Geometry check sheet. Reference: the model listing, model coordinates, mm. Face numbers are marked on the shaded views. Give positions to 0.01 mm unless a question says otherwise; leave off trailing zeros. Order: outer loops, then holes, each group sorted by start corner. A loop starts at its lowest first (then second) coordinate and runs counter-clockwise, first axis right, second up.
from build123d import *

# Parameters (mm, degrees)
SKETCH_1_R          = 53
SKETCH_1_R_2        = 45
EXTRUDE_1_DEPTH     = 8
SKETCH_2_R          = 50.25
SKETCH_2_R_2        = 46.75
CUT_EXTRUDE_1_DEPTH = 1
CUT_EXTRUDE_START   = -7
SKETCH_2_2_R        = 50.25
SKETCH_2_2_R_2      = 46.75
CUT_EXTRUDE_2_DEPTH = 1


with BuildPart() as part:
    # 草图1 → 凸台-拉伸1 (new body)
    with BuildSketch(Plane(origin=(0, 0, 0), x_dir=(1, 0, 0), z_dir=(0, 1, 0))):
        with Locations(Location((0, 0, 0), (0, 0, 270))):
            Circle(SKETCH_1_R)
        with Locations(Location((0, 0, 0), (0, 0, 270))):
            Circle(SKETCH_1_R_2, mode=Mode.SUBTRACT)
    extrude(amount=EXTRUDE_1_DEPTH)

    # 草图2 → 切除-拉伸1 (cut)
    with BuildSketch(Plane(origin=(0, 8, 0), x_dir=(1, 0, 0), z_dir=(0, 1, 0))):
        with Locations(Location((0, 0, 0), (0, 0, 270))):
            Circle(SKETCH_2_R)
        with Locations(Location((0, 0, 0), (0, 0, 270))):
            Circle(SKETCH_2_R_2, mode=Mode.SUBTRACT)
    extrude(amount=-CUT_EXTRUDE_1_DEPTH, mode=Mode.SUBTRACT)

    # 草图2<2> → 切除-拉伸2 (cut)
    with BuildSketch(Plane(origin=(0, 8, 0), x_dir=(1, 0, 0), z_dir=(0, 1, 0)).offset(CUT_EXTRUDE_START)):
        with Locations(Location((0, 0, 0), (0, 0, 270))):
            Circle(SKETCH_2_2_R)
        with Locations(Location((0, 0, 0), (0, 0, 270))):
            Circle(SKETCH_2_2_R_2, mode=Mode.SUBTRACT)
    extrude(amount=-CUT_EXTRUDE_2_DEPTH, mode=Mode.SUBTRACT)


solid = part.part
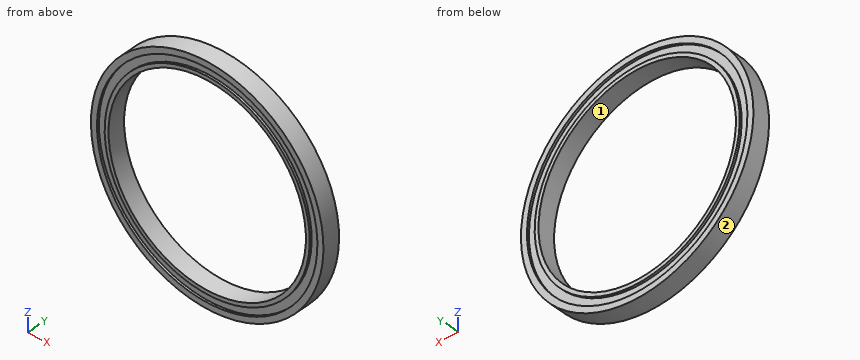
Item 1: Sectioned sample at C-C (y = 2.75). Enter the section's corners in (x, z), and give its area (3 significant figures).
Reported:
outline: circle Ø106 at (0, 0); hole circle Ø90 at (0, 0)
area: 2,460 mm2
Item 2: Sectioned sample at B-B (z = -43). Enter the section's corners in (x, y).
Reported:
outline: (-30.98, 0) - (-26, 0) - (-26, 1) - (-18.35, 1) - (-18.35, 0) - (-13.27, 0) - (-13.27, 8) - (-18.35, 8) - (-18.35, 7) - (-26, 7) - (-26, 8) - (-30.98, 8) - close; (13.27, 0) - (18.35, 0) - (18.35, 1) - (26, 1) - (26, 0) - (30.98, 0) - (30.98, 8) - (26, 8) - (26, 7) - (18.35, 7) - (18.35, 8) - (13.27, 8) - close
Item 3: Draft check along X on the marked faces 1 and 2. Enter one of: released by +X, released by -X, zero draft, split by the parting line, or undercut.
Reported:
face 1: undercut
face 2: split by the parting line
Item 4: Scan lines: L1, parallel to X at y = 0.6, z = 0; L2, parallel to X at y = 6, z = 0; L3, parallel to X at y = 7.75, z = -29.5. Record each from-to range of solid material in increasing order.
Reported:
L1: x = -53 to -50.25, -46.75 to -45, 45 to 46.75, 50.25 to 53
L2: x = -53 to -45, 45 to 53
L3: x = -44.03 to -40.68, -36.27 to -33.98, 33.98 to 36.27, 40.68 to 44.03
Item 5: Sectioned sample at A-A (x = 0). Enter the section's corners in (y, z).
Reported:
outline: (0, -53) - (8, -53) - (8, -50.25) - (7, -50.25) - (7, -46.75) - (8, -46.75) - (8, -45) - (0, -45) - (0, -46.75) - (1, -46.75) - (1, -50.25) - (0, -50.25) - close; (0, 45) - (8, 45) - (8, 46.75) - (7, 46.75) - (7, 50.25) - (8, 50.25) - (8, 53) - (0, 53) - (0, 50.25) - (1, 50.25) - (1, 46.75) - (0, 46.75) - close
Item 6: Gauge pin test, flat ends, axial feed: pin 1 (1.5 mm diameter, centred on x = 12, y = 1.5, fed in from +Z); pin 2 (12 mm diameter, centred on x = -23.5, z = 26, fed in from -Y); pin 3 (1 mm diameter, centred on y = 4, z = 4.5, fed in from +X); pin 4 (4 mm diameter, centred on y = 5.5, z = -35.5, fed in from -X). Record the tip position at first contact, or that the pin passes through.
Reported:
pin 1: stops at z = 51.79
pin 2: passes through
pin 3: stops at x = 52.85
pin 4: stops at x = -41.07
